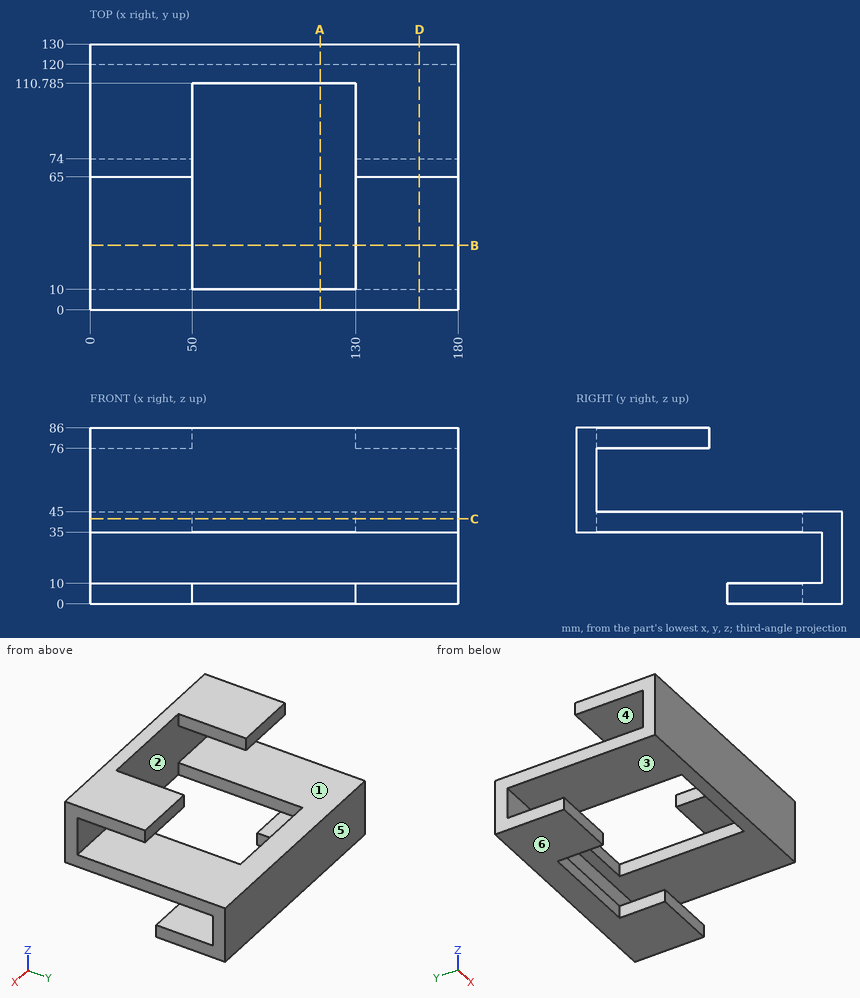
Could you check a few things on this drawing? It's one solid part, dimensions in mm from its lowest x, y, z. A direction names the side the tool comes from. Round coordinates to 2 decimals unless told otherwise and drop trailing zeros. Order: outer loops, then holes, each group sorted by start corner. A loop starts at its lowest first (then second) coordinate and runs counter-clockwise, first axis right, second up.
(1) Imagine slicing it at C-C (z = 41.5). Write out the boundary of the cut face in (x, y) (1 decimal).
Response values:
outline: (0, 0) - (180, 0) - (180, 130) - (0, 130) - close; hole (50, 10) - (130, 10) - (130, 110.8) - (50, 110.8) - close
(2) Which directions (+Z, -Z, +X, -X, +Y, -Y) give clear straight access to the entire face, cutting with the end or side of a thin tool? Please do the marked faces 1, 2 and 3.
Response values:
face 1: +X, -X, +Y
face 2: none
face 3: +X, -X, -Y
(3) Imagine slicing it at B-B (y = 31.5). Write out the boundary of the cut face in (x, z), plus the area to 3 significant figures.
Response values:
outline: (0, 35) - (50, 35) - (50, 45) - (0, 45) - close; (0, 76) - (50, 76) - (50, 86) - (0, 86) - close; (130, 35) - (180, 35) - (180, 45) - (130, 45) - close; (130, 76) - (180, 76) - (180, 86) - (130, 86) - close
area: 2,000 mm2
(4) If we mould it in two halves opening along Z, with no side actions, what happens to the marked faces 4, 5 and 6? For each: released by +Z, released by -Z, zero draft, split by the parting line, or undercut.
Response values:
face 4: undercut
face 5: zero draft
face 6: released by -Z
(5) Imagine slicing it at A-A (x = 112.5). Write out the boundary of the cut face in (y, z) (1 decimal).
Response values:
outline: (0, 35) - (10, 35) - (10, 86) - (0, 86) - close; (110.8, 0) - (130, 0) - (130, 45) - (110.8, 45) - (110.8, 35) - (120, 35) - (120, 10) - (110.8, 10) - close
(6) I'm going to push flat-ended pins straight in: pin 1 (12 mm diameter, centred on y = 22.5, z = 54, fed in from +X); pin 2 (23 mm diameter, centred on x = 125.5, y = 88.5, fed in from +Z); pin 3 (8 mm diameter, centred on x = 150, z = 3, fed in from -Y); pin 4 (3 mm diameter, centred on x = 81.5, z = 27, fed in from -Y). Where does each tip first touch, or does it pass through?
Response values:
pin 1: passes through
pin 2: stops at z = 45
pin 3: stops at y = 74
pin 4: stops at y = 120
(7) Imagine slicing it at D-D (x = 161). Write out the boundary of the cut face in (y, z).
Response values:
outline: (0, 35) - (120, 35) - (120, 10) - (74, 10) - (74, 0) - (130, 0) - (130, 45) - (10, 45) - (10, 76) - (65, 76) - (65, 86) - (0, 86) - close
(8) Please list where these lines run through material, in increasing order: line 1 along Z through (x, y) = (20, 22); line 2 along Z through (x, y) = (139.5, 83); line 3 along X through (y, z) = (23, 37.5).
Response values:
line 1: z = 35 to 45, 76 to 86
line 2: z = 0 to 10, 35 to 45
line 3: x = 0 to 50, 130 to 180
